Model file for the job. Use its own axes, mm. Face numbers are marked on the shaded views. A direction names the side the tool comes from. Give positions to 0.01 mm unless a question says otherwise; leave off trailing zeros. Write each loop counter-clockwise with the first axis right and the second up, starting at its lowest first coordinate (ties: lowest second). Pieces come first, ordered by that corner, then holes. Notation, with made-up numbers: M -11.5,-13 L 6.5,-13 A20 ccw 6.5,16 Z; hole C -22,37.25 d6. An arc over 180 degrees is marked long. Answer as a JSON object with one key per item and string values. Group by question number.
```python
from build123d import *

# Parameters (mm, degrees)
ESQUISSE1_W                                       = 12
ESQUISSE1_H                                       = 40
BOSS_EXTRU_1_DEPTH                                = 4
ESQUISSE2_W                                       = 12
ESQUISSE2_H                                       = 6
BOSS_EXTRU_2_DEPTH                                = 10
ESQUISSE4_W                                       = 12
ESQUISSE4_H                                       = 5
BOSS_EXTRU_3_DEPTH                                = 6
ESQUISSE5_R                                       = 0.95
ENL_V_MAT_EXTRU_2_DEPTH                           = 5
ESQUISSE6_W                                       = 10
ESQUISSE6_H                                       = 40
BOSS_EXTRU_4_DEPTH                                = 5
ESQUISSE7_R                                       = 2
ENL_V_MAT_EXTRU_3_DEPTH                           = 2
CHAMBRAGE_POUR_VIS_SIX_PANS_CREUX_M21_D           = 2.4
CHAMBRAGE_POUR_VIS_SIX_PANS_CREUX_M21_DEPTH       = 6
CHAMBRAGE_POUR_VIS_SIX_PANS_CREUX_M21_CBORE_D     = 4.4
CHAMBRAGE_POUR_VIS_SIX_PANS_CREUX_M21_CBORE_DEPTH = 2.4
ESQUISSE15_W                                      = 12
ESQUISSE15_H                                      = 2.3
ESQUISSE15_W_2                                    = 2.3
ESQUISSE15_H_2                                    = 15
ENL_V_MAT_EXTRU_4_DEPTH                           = 1.2


with BuildPart() as part:
    # Esquisse1 → Boss.-Extru.1 (new body)
    with BuildSketch(Plane.XY):
        with Locations((4, 2.5)):
            Rectangle(ESQUISSE1_W, ESQUISSE1_H)
    extrude(amount=BOSS_EXTRU_1_DEPTH)

    # Esquisse2 → Boss.-Extru.2 (add)
    with BuildSketch(Plane(origin=(0, 0, 0), x_dir=(-1, 0, 0), z_dir=(0, 0, -1))):
        with Locations((-4, -14.5)):
            Rectangle(ESQUISSE2_W, ESQUISSE2_H)
    boss_extru_2 = extrude(amount=BOSS_EXTRU_2_DEPTH)

    # Symétrie1: Boss.-Extru.2 across plane
    add(boss_extru_2.mirror(Plane.ZX))

    # Esquisse4 → Boss.-Extru.3 (add)
    with BuildSketch(Plane.XY.offset(4)):
        with Locations((4, 20)):
            Rectangle(ESQUISSE4_W, ESQUISSE4_H)
        with Locations((4, -15)):
            Rectangle(ESQUISSE4_W, ESQUISSE4_H)
    extrude(amount=BOSS_EXTRU_3_DEPTH)

    # Esquisse5 → Enlèv. mat.-Extru.2 (cut)
    with BuildSketch(Plane.XY.offset(10)):
        with Locations((4, -15)):
            Circle(ESQUISSE5_R)
        with Locations(Location((4, 20, 0), (0, 0, 180))):
            Circle(ESQUISSE5_R)
    extrude(amount=-ENL_V_MAT_EXTRU_2_DEPTH, mode=Mode.SUBTRACT)

    # Esquisse6 → Boss.-Extru.4 (add)
    with BuildSketch(Plane.ZY.offset(2)):
        with Locations((5, 2.5)):
            Rectangle(ESQUISSE6_W, ESQUISSE6_H)
    extrude(amount=BOSS_EXTRU_4_DEPTH)

    # Esquisse7 → Enlèv. mat.-Extru.3 (cut)
    with BuildSketch(Plane(origin=(-2, 0, 0), x_dir=(0, 0, -1), z_dir=(1, 0, 0))):
        with Locations(Location((-7, -6, 0), (0, 0, 90))):
            Circle(ESQUISSE7_R)
    extrude(amount=-ENL_V_MAT_EXTRU_3_DEPTH, mode=Mode.SUBTRACT)

    # Chambrage pour vis à six pans creux M21
    with Locations(Plane(origin=(0, -17.5, 0), x_dir=(-1, 0, 0), z_dir=(0, -1, 0))):
        with Locations((-5, 5)):
            chambrage_pour_vis_six_pans_creux_m21 = CounterBoreHole(CHAMBRAGE_POUR_VIS_SIX_PANS_CREUX_M21_D / 2, CHAMBRAGE_POUR_VIS_SIX_PANS_CREUX_M21_CBORE_D / 2, CHAMBRAGE_POUR_VIS_SIX_PANS_CREUX_M21_CBORE_DEPTH, depth=CHAMBRAGE_POUR_VIS_SIX_PANS_CREUX_M21_DEPTH)

    # Symétrie2: Chambrage pour vis à six pans creux M21 across plane
    add(chambrage_pour_vis_six_pans_creux_m21.mirror(Plane.ZX), mode=Mode.SUBTRACT)

    # Esquisse15 → Enlèv. mat.-Extru.4 (cut)
    with BuildSketch(Plane.XY.offset(4)):
        with Locations((4, -6)):
            Rectangle(ESQUISSE15_W, ESQUISSE15_H)
        with Locations((4, 10)):
            Rectangle(ESQUISSE15_W_2, ESQUISSE15_H_2)
    extrude(amount=-ENL_V_MAT_EXTRU_4_DEPTH, mode=Mode.SUBTRACT)


solid = part.part
```
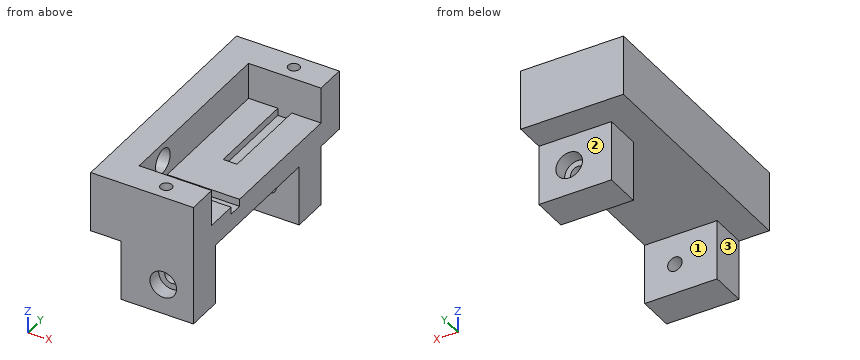
Q1. Slice it at C-C, the plane z = 4.5. Write the cut outline in (x, y), then the cut area to 3 significant figures.
Q2. Slice it at D-D, the plane x = 2. Write the cut outline in (y, z).
Q3. Slice it at A-A, the plane z = 7. Write the cut outline in (x, y).
Q4. Wall check: L1, parallel to Y at x = 4, z = 7.15; L2, parallel to Z at x = 5, y = -15.85; L3, parallel to X at y = -13.9, z = -5. Give the ranges that are in metal, low to high.
Q5. Drop flat-ended pins along their axis: P1, Ø1.2, axis at x = 4, y = 11.5, coming from the +Z side; P2, Ø3, axis at x = 2.5, y = -6, coming from the -Z side; P3, Ø2, axis at x = 5.5, z = -4.5, coming from the -Y side. Give the stop position or say it passes through.
Q6. 3-axis set-ups, long thin cutter, end or side, ignore diameter. For the marked faces 1, 2 and 3: which of +Z, -Z, +X, -X, +Y, -Y reach the whole face in a straight line?
Q7. Slice it at B-B, the plane z = -5. Write the cut outline in (x, y).
Solved:
{
 "1": {"outline": "M -7,-17.5 L 10,-17.5 L 10,-12.5 L -2,-12.5 L -2,17.5 L 10,17.5 L 10,22.5 L -7,22.5 Z", "area": "320 mm²"},
 "2": {"outline": "M -17.5,-10 L -11.5,-10 L -11.5,0 L 11.5,0 L 11.5,-10 L 17.5,-10 L 17.5,0 L 22.5,0 L 22.5,10 L 17.5,10 L 17.5,4 L -4.85,4 L -4.85,2.8 L -7.15,2.8 L -7.15,4 L -12.5,4 L -12.5,10 L -17.5,10 Z"},
 "3": {"outline": "M -7,-17.5 L 10,-17.5 L 10,-12.5 L -2,-12.5 L -2,-8 L -4,-8 L -4,-4 L -2,-4 L -2,17.5 L 10,17.5 L 10,22.5 L -7,22.5 Z; hole C 4,-15 d1.9; hole C 4,20 d1.9"},
 "4": {"L1": "y = -17.5 to -15.95, -14.05 to -12.5, 17.5 to 19.05, 20.95 to 22.5", "L2": "z = -10 to -7.2, -2.8 to 10", "L3": "x = -2 to 3.8, 6.2 to 10"},
 "5": {"P1": "stops at z = 2.8", "P2": "stops at z = 0", "P3": "stops at y = -15.1"},
 "6": {"face 1": "-Z, +X, -X", "face 2": "-Z, +X, -X, +Y", "face 3": "-Z, -X, +Y, -Y"},
 "7": {"outline": "M -2,-17.5 L 2.8,-17.5 L 2.8,-15.1 L 3.8,-15.1 L 3.8,-11.5 L -2,-11.5 Z; M -2,11.5 L 3.8,11.5 L 3.8,15.1 L 2.8,15.1 L 2.8,17.5 L -2,17.5 Z; M 6.2,-15.1 L 7.2,-15.1 L 7.2,-17.5 L 10,-17.5 L 10,-11.5 L 6.2,-11.5 Z; M 6.2,11.5 L 10,11.5 L 10,17.5 L 7.2,17.5 L 7.2,15.1 L 6.2,15.1 Z"}
}
